Read the model definition and answer for the solid it produces. Units are mm, in the model's axes. A direction names the side the tool comes from. Round coordinates to 2 decimals unless told otherwise and drop trailing zeros. Loops run counter-clockwise (first coordinate to the right, second up) from the corner with the lowest first, then second, coordinate; pieces in that order, holes last. Notation, with made-up numbers: (47.25, 15) - (63.25, 15) arc R8 cw to (63.25, 30) - close; hole circle Ø5 at (56.25, 83). An arc over 180 degrees is marked (long way). Answer as CSV lines item,"result".
```python
from build123d import *

# Parameters (mm, degrees)
SKETCH1_R           = 14
BOSS_EXTRUDE1_DEPTH = 17.5
CHAMFER1_SIZE       = 2.54
CHAMFER1_SIZE2      = 4.399409051
SKETCH2_R           = 1.5875
BOSS_EXTRUDE2_DEPTH = 10.1


with BuildPart() as part:
    # Sketch1 → Boss-Extrude1 (new body, symmetric)
    with BuildSketch(Plane(origin=(0, 0, 0), x_dir=(1, 0, 0), z_dir=(0, 1, 0))):
        Circle(SKETCH1_R)
    extrude(amount=BOSS_EXTRUDE1_DEPTH, both=True)

    # Chamfer1
    chamfer1_edges = [part.edges().sort_by_distance(p)[0] for p in [
        (-14, 17.5, 0),
    ]]
    chamfer1_side = [part.faces().sort_by_distance(p)[0] for p in [
        (-14, 0, 0),
    ]]
    chamfer(chamfer1_edges, length=CHAMFER1_SIZE, length2=CHAMFER1_SIZE2, reference=chamfer1_side[0])

    # Sketch2 → Boss-Extrude2 (add)
    with BuildSketch(Plane.XZ.offset(17.5)):
        Circle(SKETCH2_R)
    extrude(amount=BOSS_EXTRUDE2_DEPTH)


solid = part.part
```
1) A tool of negligible diameter and unlimited length cuts with its end or side. For faces 1 (the face through (0, -27.6, 0)), 2 (the face through (-0.34, -22.48, -1.55)), from which of +Z, -Z, +X, -X, +Y, -Y can it reach the whole face along a straight path? Write none if from no direction.
Entries:
face 1,"+Z, -Z, +X, -X, -Y"
face 2,"-Y"
2) Each of these flat-tipped pins is pushed along its axis until it touches: P1, Ø1, axis at x = 5, y = 4, coming from the +Z side; P2, Ø2, axis at x = 10, z = 8.5, coming from the -Y side; P3, Ø8, axis at x = 5.5, y = 4, coming from the +Z side. Where does it stop, or does it pass through?
Entries:
P1,"stops at z = 13.26"
P2,"stops at y = -17.5"
P3,"stops at z = 13.92"
3) A cutting plane is placed at C-C, the plane y = 2.5. Determine the outline of the cut face in (x, z).
Entries:
outline,"circle Ø28 at (0, 0)"
4) A cutting plane is placed at B-B, the plane z = 0. Determine the outline of the cut face in (x, y), plus the area to 3 significant figures.
Entries:
outline,"(-14, -17.5) - (-1.59, -17.5) - (-1.59, -27.6) - (1.59, -27.6) - (1.59, -17.5) - (14, -17.5) - (14, 14.96) - (9.6, 17.5) - (-9.6, 17.5) - (-14, 14.96) - close"
area,"1,000 mm^2"
5) A cutting plane is placed at A-A, the plane x = 0. Determine the outline of the cut face in (y, z).
Entries:
outline,"(-27.6, -1.59) - (-17.5, -1.59) - (-17.5, -14) - (14.96, -14) - (17.5, -9.6) - (17.5, 9.6) - (14.96, 14) - (-17.5, 14) - (-17.5, 1.59) - (-27.6, 1.59) - close"
6) Find the intervals of material crossed by line 1 (Y direction, x = 7.5, z = 6); line 2 (Z direction, x = 0.5, y = 11); line 3 (X direction, y = 13.5, z = -10.5), in increasing order.
Entries:
line 1,"y = -17.5 to 17.5"
line 2,"z = -13.99 to 13.99"
line 3,"x = -9.26 to 9.26"
